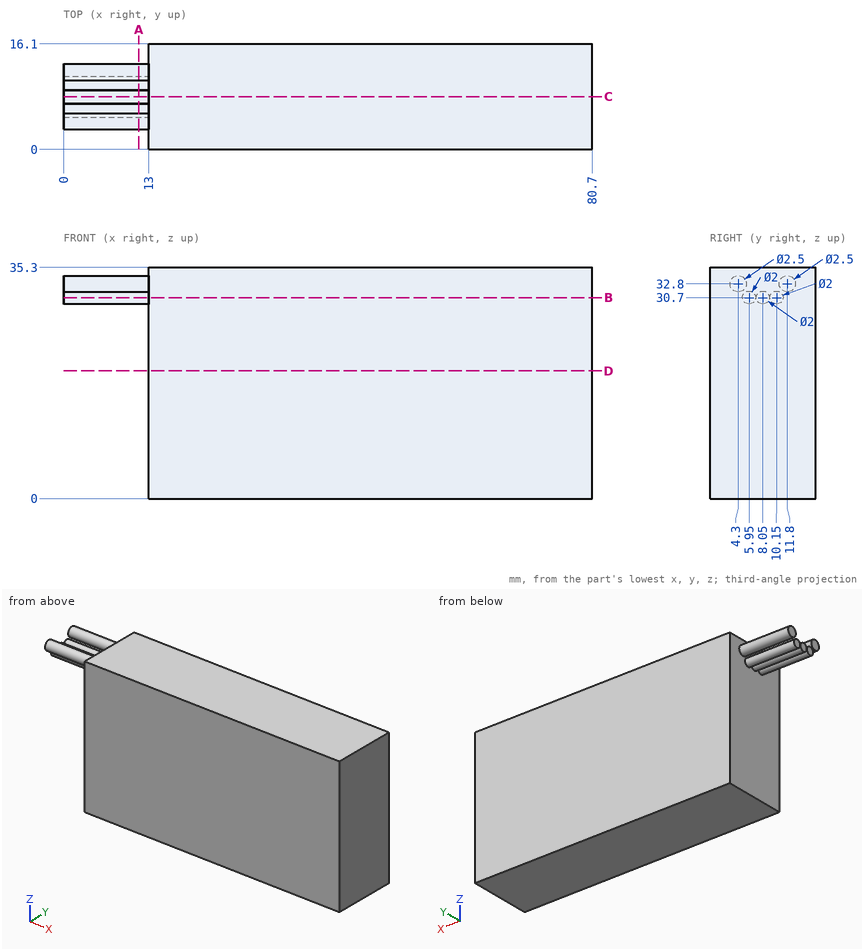
Input: dimensioned drawing with shaded views. Units: mm. Origin: part minimum x, y, z. Coordinates: 2 decimals unless noted, no trailing zeros. Loops run counter-clockwise (first coordinate to the right, second up) from the corner with the lowest first, then second, coordinate; pieces in that order, holes last. Notation, with made-up numbers: M 19,25.25 L 28,25.25 A20 cw 28,31.25 Z; hole C 4.25,29 d6. An arc over 180 degrees is marked long. Use a Markdown table: item, result. Add a question column.
Q1. First-contact query: pin 1 (3 mm diameter, centred on x = 50, z = 9, fed in from -Y); pin 2 (1 mm diameter, centred on y = 7, z = 21, fed in from -X). Flat tips, straight axial feed; report the tip coordinate or a pass-through.
Q2. Section query C-C, the plane y = 8.05. Return loops of the section in (x, z), and give its area (3 significant figures).
Q3. Material intervals for L1, parallel to X at y = 9, z = 23; L2, parallel to Z at x = 5, y = 8.75; L3, parallel to Z at x = 5, y = 11.5, sorted ascending.
Q4. Section query D-D, the plane z = 19.5. Return loops of the section in (x, y).
Q5. Section query A-A, the plane x = 11.5. Return loops of the section in (y, z).
Q6. Section query B-B, the plane z = 30.7. Return loops of the section in (x, y), and give its area (3 significant figures).
Result:
| question | item | result |
|---|---|---|
| 1 | pin 1 | stops at y = 0 |
| 1 | pin 2 | stops at x = 13 |
| 2 | outline | M 0,29.7 L 13,29.7 L 13,0 L 80.7,0 L 80.7,35.3 L 13,35.3 L 13,31.7 L 0,31.7 Z |
| 2 | area | 2,420 mm2 |
| 3 | L1 | x = 13 to 80.7 |
| 3 | L2 | z = 29.99 to 31.41 |
| 3 | L3 | z = 31.59 to 34.01 |
| 4 | outline | M 13,0 L 80.7,0 L 80.7,16.1 L 13,16.1 Z |
| 5 | outline | C 4.3,32.8 d2.5; C 5.95,30.7 d2; C 8.05,30.7 d2; C 10.15,30.7 d2; C 11.8,32.8 d2.5 |
| 6 | outline | M 0,4.95 L 13,4.95 L 13,0 L 80.7,0 L 80.7,16.1 L 13,16.1 L 13,11.15 L 0,11.15 L 0,9.15 L 13,9.15 L 13,9.05 L 0,9.05 L 0,7.05 L 13,7.05 L 13,6.95 L 0,6.95 Z |
| 6 | area | 1,170 mm2 |
